CAD build for the part. Positions are in the model's coordinates, mm. Face numbers are marked on the shaded views. A direction names the side the tool comes from. Coordinates: 2 decimals unless noted, no trailing zeros. Write each loop counter-clockwise with the first axis right and the second up, starting at its lowest first coordinate (ties: lowest second). Pieces come first, ordered by that corner, then holes.
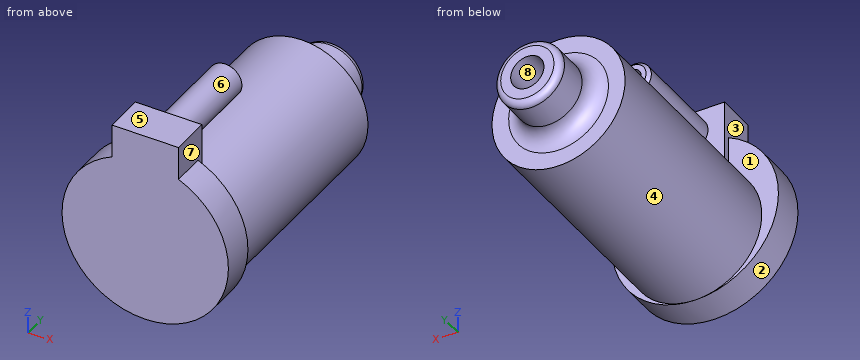
```python
from build123d import *

# Parameters (mm, degrees)
SKETCH_1_R          = 20
EXTRUDE_1_DEPTH     = 80
SKETCH_2_R          = 10
EXTRUDE_2_DEPTH     = 16
SKETCH_3_R          = 25
EXTRUDE_3_DEPTH     = 10
SKETCH_4_W          = 20
SKETCH_4_H          = 38
EXTRUDE_4_DEPTH     = 12
SKETCH_5_R          = 5
EXTRUDE_5_DEPTH     = 30
FILLET_1_R          = 5
FILLET_2_R          = 2
SKETCH_6_R          = 5
CUT_EXTRUDE_1_DEPTH = 30
SKETCH_7_R          = 2.5
CUT_EXTRUDE_2_DEPTH = 30
CHAMFER_1_SIZE      = 1


with BuildPart() as part:
    # Эскиз1 → Бобышка-Вытянуть1 (new body)
    with BuildSketch(Plane(origin=(0, 0, 0), x_dir=(1, 0, 0), z_dir=(0, 1, 0))):
        with Locations(Location((0, 0, 0), (0, 0, 270))):
            Circle(SKETCH_1_R)
    extrude(amount=EXTRUDE_1_DEPTH)

    # Эскиз2 → Бобышка-Вытянуть2 (add)
    with BuildSketch(Plane(origin=(0, 80, 0), x_dir=(1, 0, 0), z_dir=(0, 1, 0))):
        with Locations(Location((0, 0, 0), (0, 0, 270))):
            Circle(SKETCH_2_R)
    extrude(amount=EXTRUDE_2_DEPTH)

    # Эскиз3 → Бобышка-Вытянуть3 (add)
    with BuildSketch(Plane.XZ):
        with Locations(Location((0, 5, 0), (0, 0, 270))):
            Circle(SKETCH_3_R)
    extrude(amount=-EXTRUDE_3_DEPTH)

    # Эскиз4 → Бобышка-Вытянуть4 (add)
    with BuildSketch(Plane.XZ):
        with Locations((0, 19)):
            Rectangle(SKETCH_4_W, SKETCH_4_H)
    extrude(amount=-EXTRUDE_4_DEPTH)

    # Эскиз5 → Бобышка-Вытянуть5 (add)
    with BuildSketch(Plane(origin=(0, 12, 0), x_dir=(1, 0, 0), z_dir=(0, 1, 0))):
        with Locations(Location((0, -31, 0), (0, 0, 90))):
            Circle(SKETCH_5_R)
    extrude(amount=EXTRUDE_5_DEPTH)

    # Скругление1
    fillet_1_edges = [part.edges().sort_by_distance(p)[0] for p in [
        (0, 80, -10),
    ]]
    fillet(fillet_1_edges, radius=FILLET_1_R)

    # Скругление2
    fillet_2_edges = [part.edges().sort_by_distance(p)[0] for p in [
        (0, 96, -10),
    ]]
    fillet(fillet_2_edges, radius=FILLET_2_R)

    # Эскиз6 → Вырез-Вытянуть1 (cut)
    with BuildSketch(Plane(origin=(0, 96, 0), x_dir=(1, 0, 0), z_dir=(0, 1, 0))):
        with Locations(Location((0, 0, 0), (0, 0, 270))):
            Circle(SKETCH_6_R)
    extrude(amount=-CUT_EXTRUDE_1_DEPTH, mode=Mode.SUBTRACT)

    # Эскиз7 → Вырез-Вытянуть2 (cut)
    with BuildSketch(Plane(origin=(0, 42, 0), x_dir=(1, 0, 0), z_dir=(0, 1, 0))):
        with Locations(Location((0, -31, 0), (0, 0, 270))):
            Circle(SKETCH_7_R)
    extrude(amount=-CUT_EXTRUDE_2_DEPTH, mode=Mode.SUBTRACT)

    # Фаска1
    chamfer_1_edges = [part.edges().sort_by_distance(p)[0] for p in [
        (0, 42, 36),
    ]]
    chamfer(chamfer_1_edges, length=CHAMFER_1_SIZE)


solid = part.part
```
Item 1: Saw through at C-C, the plane x = 18. Write the cut outline in (y, z), and give its area (3 significant figures).
Item 2: Saw through at D-D, the plane y = 83.5. Write the cut outline in (x, z).
Item 3: Saw through at A-A, the plane z = 31. Write the cut outline in (x, y).
Item 4: Which spindle directions (+Z, -Z, +X, -X, +Y, -Y) get a long thin tool onto all of the face, cutting with end or side? Do the marked faces 1, 2, 3 and 4. Say none if no direction does.
Item 5: Saw through at B-B, the plane y = 26. Write the cut outline in (x, z), and give its area (3 significant figures).
Item 6: Flat gauge pins, fed straight in: pin 1 Ø10 at (x, z) = (1.5, 29) entering from +Y; pin 2 Ø3.5 at (y, z) = (7, 32.5) entering from -X; pin 3 Ø1.5 at (x, y) = (-1.5, 82) entering from -Z. Where does each tip first touch, or does it go through?
Item 7: Wall check: line 1 along X through (y, z) = (85, 0); line 2 along X through (y, z) = (27.5, 31); line 3 along Y through (x, z) = (16, 15). Give the ranges that are in metal, low to high.
Item 8: Two-plate mould, pull along X, no slides. Class the marked faces 5, 6, 7 and 8: +X half, -X half, draft (parallel to the pull), parting line (faces both ways), or undercut.
Working result:
1. outline: (0, -12.35) - (10, -12.35) - (10, -8.72) - (80, -8.72) - (80, 8.72) - (10, 8.72) - (10, 22.35) - (0, 22.35) - close
1. area: 1,570 mm2
2. outline: circle Ø20.46 at (0, 0); hole circle Ø10 at (0, 0)
3. outline: (-10, 0) - (10, 0) - (10, 12) - (5, 12) - (5, 41) - (4, 42) - (2.5, 42) - (2.5, 12) - (-2.5, 12) - (-2.5, 42) - (-4, 42) - (-5, 41) - (-5, 12) - (-10, 12) - close
4. face 1: -X, +Y
4. face 2: +Y, -Y
4. face 3: +Z, -X, +Y
4. face 4: +Y
5. outline: circle Ø40 at (0, 0); circle Ø10 at (0, 31); hole circle Ø5 at (0, 31)
5. area: 1,320 mm2
6. pin 1: stops at y = 42
6. pin 2: stops at x = -10
6. pin 3: stops at z = -11.6
7. line 1: x = -10 to -5, 5 to 10
7. line 2: x = -5 to -2.5, 2.5 to 5
7. line 3: y = 0 to 10
8. face 5: draft
8. face 6: parting line
8. face 7: +X half
8. face 8: undercut
